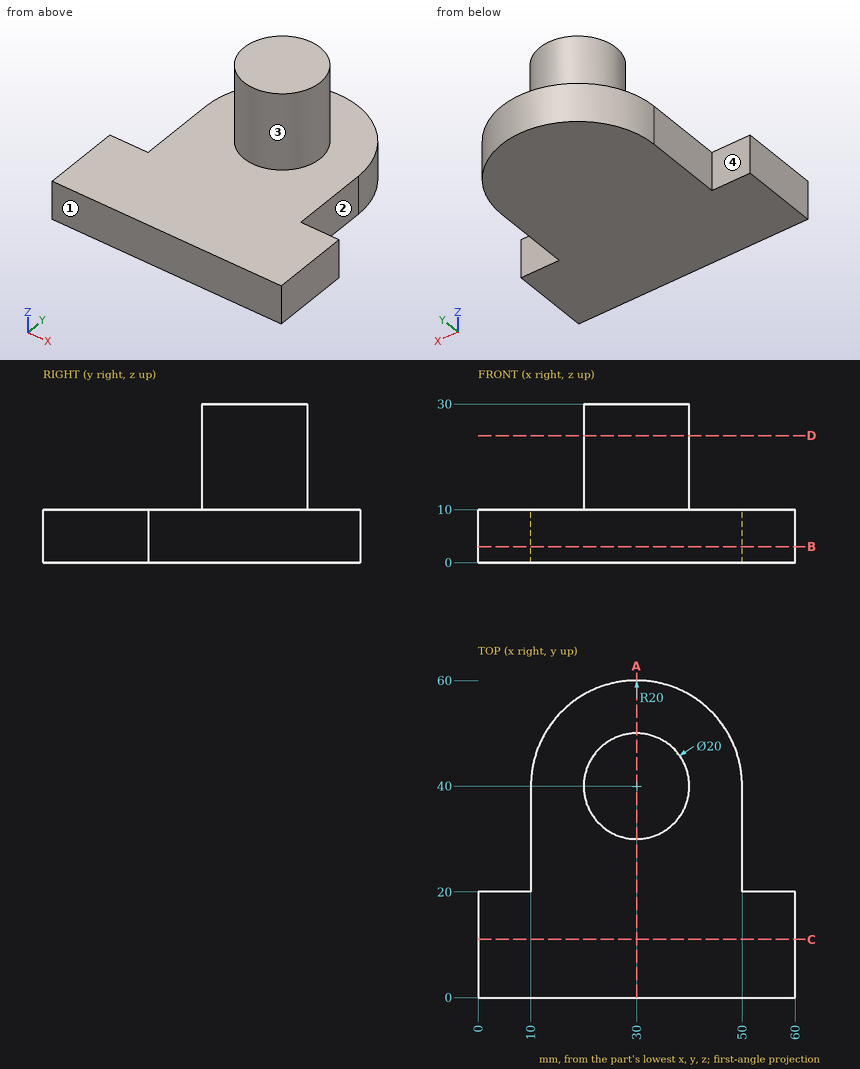
For this review, use the dimensioned drawing (mm, ordinates from the lowest corner) and the shaded views. A direction names the side the tool comes from. Give positions to 0.01 mm unless a question says otherwise; leave off trailing zeros. Write each loop counter-clockwise with the first axis right and the second up, starting at its lowest first coordinate (ties: lowest second). Pieces come first, ordered by that corner, then holes.
(1) Consider section B-B, the plane z = 3. Give the boundary of the cut face in (x, y), and give its area (3 significant figures).
(2) Tool access review of the marked faces 1, 2, 3 and 4: name each direction out of +Z, -Z, +X, -X, +Y, -Y from which nothing blocks a thin tool from reaching the whole face with its end or side.
(3) To check wall thickness, follow L1, parallel to Z at x = 50.5, y = 11.5; L2, parallel to Y at x = 27.5, z = 24.25; L3, parallel to X at y = 42, z = 19.5. State the ranges of each line that lie inside material, in increasing order.
(4) For P1, Ø11, axis at y = 31, z = 3.5, coming from the -X side; P2, Ø12, axis at x = 40, y = 24, coming from the +Z side; P3, Ø8, axis at x = 54.5, z = 3.5, coming from the +Y side; P4, Ø10, axis at y = 7, z = 18, coming from the +X side, all flat-tipped, find the tip position at first contact; note any pin that passes through.
(5) Consider section D-D, the plane z = 24. Give the boundary of the cut face in (x, y).
(6) Consider section C-C, the plane y = 11. Give the boundary of the cut face in (x, z), and give its area (3 significant figures).
(7) Consider section A-A, the plane x = 30. Give the boundary of the cut face in (y, z), and give its area (3 significant figures).
Returned:
1. outline: (0, 0) - (60, 0) - (60, 20) - (50, 20) - (50, 40) arc R20 ccw to (10, 40) - (10, 20) - (0, 20) - close
1. area: 2,630 mm2
2. face 1: +Z, -Z, +X, -X, -Y
2. face 2: +Z, -Z, +X, +Y
2. face 3: +Z
2. face 4: +Z, -Z, -X, +Y
3. L1: z = 0 to 10
3. L2: y = 30.32 to 49.68
3. L3: x = 20.2 to 39.8
4. P1: stops at x = 10
4. P2: stops at z = 10
4. P3: stops at y = 20
4. P4: passes through
5. outline: circle Ø20 at (30, 40)
6. outline: (0, 0) - (60, 0) - (60, 10) - (0, 10) - close
6. area: 600 mm2
7. outline: (0, 0) - (60, 0) - (60, 10) - (50, 10) - (50, 30) - (30, 30) - (30, 10) - (0, 10) - close
7. area: 1,000 mm2
